from build123d import *

# Parameters (mm, degrees)
SKETCH1_R               = 4.725
BOSS_EXTRUDE1_DEPTH     = 6.56
SKETCH5_R               = 10
BOSS_EXTRUDE3_DEPTH     = 15
CUT_EXTRUDE1_DEPTH      = 5
CUT_EXTRUDE1_DEPTH_BACK = 15
SKETCH4_W               = 2
SKETCH4_H               = 12
CUT_EXTRUDE2_DEPTH      = 10
CUT_EXTRUDE3_REACH      = 31.813
SKETCH6_R               = 2
SKETCH7_R               = 1.75
CUT_EXTRUDE4_DEPTH      = 26.784367357


with BuildPart() as part:
    # Sketch1 → Boss-Extrude1 (new body)
    with BuildSketch(Plane.XY):
        Circle(SKETCH1_R)
    extrude(amount=-BOSS_EXTRUDE1_DEPTH)

    # Sketch5 → Boss-Extrude3 (add)
    with BuildSketch(Plane(origin=(0, 0, -6.56), x_dir=(-1, 0, 0), z_dir=(0, 0, -1))):
        Circle(SKETCH5_R)
    extrude(amount=BOSS_EXTRUDE3_DEPTH)

    # Sketch3 → Cut-Extrude1 (cut, two sides: drawn at the far end of the back side and taken through both)
    with BuildSketch(Plane(origin=(0, 0, 0), x_dir=(0, 0, -1), z_dir=(1, 0, 0)).offset(-CUT_EXTRUDE1_DEPTH_BACK)):
        Polygon((21.56, -5), (21.56, 5), (11.56, 7.679491924), (11.56, -7.679491924), align=None)
    extrude(amount=CUT_EXTRUDE1_DEPTH + CUT_EXTRUDE1_DEPTH_BACK, mode=Mode.SUBTRACT)

    # Sketch4 → Cut-Extrude2 (cut)
    with BuildSketch(Plane(origin=(0, 0, -21.56), x_dir=(-1, 0, 0), z_dir=(0, 0, -1))):
        with Locations((-9, 0)):
            Rectangle(SKETCH4_W, SKETCH4_H)
    extrude(amount=-CUT_EXTRUDE2_DEPTH, mode=Mode.SUBTRACT)

    # Sketch6 → Cut-Extrude3 (cut, up to next)
    with BuildSketch(Plane(origin=(8, 0, 0), x_dir=(0, 0, -1), z_dir=(1, 0, 0)), mode=Mode.PRIVATE) as cut_extrude3_sk1:
        with Locations((16.56, 0)):
            Circle(SKETCH6_R)
    cut_extrude3_tool1 = extrude(cut_extrude3_sk1.sketch, amount=-CUT_EXTRUDE3_REACH, mode=Mode.PRIVATE) & part.part
    add(cut_extrude3_tool1.solids().sort_by_distance((8, 0, -16.56))[0], mode=Mode.SUBTRACT)

    # Sketch7 → Cut-Extrude4 (cut, through all)
    with BuildSketch(Plane.XY):
        Circle(SKETCH7_R)
    extrude(amount=-CUT_EXTRUDE4_DEPTH, mode=Mode.SUBTRACT)


solid = part.part
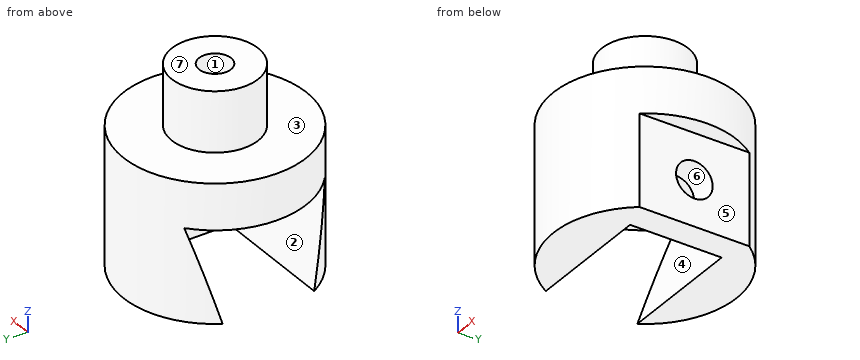
Model file for the job. Use its own axes, mm. Face numbers are marked on the shaded views. A direction names the side the tool comes from. Round coordinates to 2 decimals unless told otherwise and drop trailing zeros. Loops run counter-clockwise (first coordinate to the right, second up) from the corner with the lowest first, then second, coordinate; pieces in that order, holes last. Notation, with made-up numbers: (-34.5, 0) - (-8.5, 0) arc R23 cw to (-8.5, 28) - close; hole circle Ø11 at (-10.5, 73). An arc over 180 degrees is marked (long way). Write each question's results on one line, items separated by ' | '.
(1) Pin check, flat tips, straight feed: pin 1 (3 mm diameter, centred on x = 0, y = 0, fed in from -Z); pin 2 (1 mm diameter, centred on x = -5.5, z = -13.5, fed in from -Y); pin 3 (5 mm diameter, centred on y = -2, z = -14.5, fed in from +X); pin 4 (5 mm diameter, centred on y = 1.5, z = -14, fed in from -X). Stop position of each tip, or through.
Answer below:
pin 1: passes through | pin 2: stops at y = -8.66 | pin 3: stops at x = 8 | pin 4: stops at x = -9.95
(2) Saw through at D-D, the plane z = -10. List the corners of the cut face in (x, y).
Answer below:
outline: circle Ø20 at (0, 0); hole circle Ø3.5 at (0, 0)
(3) Mould opens along Z. For the marked faces 4, 5, 6 and 7 say: released by +Z, released by -Z, zero draft, split by the parting line, or undercut.
Answer below:
face 4: undercut | face 5: zero draft | face 6: undercut | face 7: released by +Z
(4) Saw through at A-A, the plane y = 0. List the corners of the cut face in (x, z) (3 decimals).
Answer below:
outline: (-10, -11.56) - (-1.75, -11.56) - (-1.75, 0) - (-4.725, 0) - (-4.725, -6.56) - (-10, -6.56) - close; (1.75, -11.56) - (5, -11.56) - (5, -14.56) - (8, -14.56) - (8, -11.56) - (10, -11.56) - (10, -6.56) - (4.725, -6.56) - (4.725, 0) - (1.75, 0) - close; (5, -21.56) - (8, -21.56) - (8, -18.56) - (5, -18.56) - close
(5) Wall check: L1, parallel to Y at x = 0, z = -4.75 (3 decimals); L2, parallel to Y at x = 0, z = -7.5; L3, parallel to X at y = 0, z = -12.5. Give the ranges that are in metal, low to high.
Answer below:
L1: y = -4.725 to -1.75, 1.75 to 4.725 | L2: y = -10 to -1.75, 1.75 to 10 | L3: x = 5 to 8
(6) 3-axis set-ups, long thin cutter, end or side, ignore diameter. For the marked faces 1, 2 and 3: which of +Z, -Z, +X, -X, +Y, -Y reach the whole face in a straight line?
Answer below:
face 1: +Z, -Z | face 2: -X | face 3: +Z
(7) Saw through at C-C, the plane z = -16.56. List the corners of the cut face in (x, y), then the cut area to 3 significant figures.
Answer below:
outline: (-7.73, -6.34) arc R10 ccw to (8, -6) - (8, -2) - (5, -2) - (5, -6.34) - close; (-7.73, 6.34) - (5, 6.34) - (5, 2) - (8, 2) - (8, 6) arc R10 ccw to start | area: 105 mm^2
